For this review, take the finished solid that the model builds, in its own axes (mm). A direction names the side the tool comes from. Coordinates: 2 decimals unless noted, no trailing zeros. Order: outer loops, then holes, each group sorted by start corner. A loop starts at its lowest first (then second) coordinate and runs counter-clockwise, first axis right, second up.
from build123d import *

# Parameters (mm, degrees)
SKETCH1_R               = 4
BOSS_EXTRUDE1_DEPTH     = 3
SKETCH1_3_R             = 2.5
BOSS_EXTRUDE2_DEPTH     = 13
BOSS_EXTRUDE3_DEPTH     = 1.5
CUT_EXTRUDE1_DEPTH      = 15.177446879
CUT_EXTRUDE1_DEPTH_BACK = 15.177446879
SKETCH2_W               = 10
SKETCH2_H               = 3


with BuildPart() as part:
    # Sketch1 → Boss-Extrude1 (new body)
    with BuildSketch(Plane(origin=(0, 0, 0), x_dir=(0, 0, -1), z_dir=(1, 0, 0))):
        Circle(SKETCH1_R)
    extrude(amount=BOSS_EXTRUDE1_DEPTH)

    # Sketch1<3> → Boss-Extrude2 (add)
    with BuildSketch(Plane(origin=(0, 0, 0), x_dir=(0, 0, -1), z_dir=(1, 0, 0))):
        Circle(SKETCH1_3_R)
    extrude(amount=-BOSS_EXTRUDE2_DEPTH)

    # Sketch3 → Boss-Extrude3 (add, symmetric)
    with BuildSketch(Plane(origin=(0, 0, 0), x_dir=(1, 0, 0), z_dir=(0, 1, 0))):
        with BuildLine():
            Line((-11, 2.5), (-11, -2.5))
            ThreePointArc((-11, -2.5), (-12, -3.5), (-13, -2.5))
            Line((-13, -2.5), (-13, 2.5))
            ThreePointArc((-13, 2.5), (-12, 3.5), (-11, 2.5))
        make_face()
    extrude(amount=BOSS_EXTRUDE3_DEPTH, both=True)

    # Sketch2 → Cut-Extrude1 (cut, two sides: drawn at the far end of the back side and taken through both)
    with BuildSketch(Plane(origin=(0, 0, 0), x_dir=(1, 0, 0), z_dir=(0, 1, 0)).offset(-CUT_EXTRUDE1_DEPTH_BACK)):
        with Locations((-8, 0)):
            Rectangle(SKETCH2_W, SKETCH2_H)
    extrude(amount=CUT_EXTRUDE1_DEPTH + CUT_EXTRUDE1_DEPTH_BACK, mode=Mode.SUBTRACT)


solid = part.part
1. Take a section at D-D, the plane x = 0.75. Give the boundary of the cut face in (y, z).
Answer below:
outline: circle Ø8 at (0, 0)
2. Take a section at A-A, the plane x = -12. Give the boundary of the cut face in (y, z).
Answer below:
outline: (-2, -1.5) arc R2.5 ccw to (-1.5, -2) - (-1.5, -3.5) - (1.5, -3.5) - (1.5, -2) arc R2.5 ccw to (2, -1.5) - close; (-2, 1.5) - (2, 1.5) arc R2.5 ccw to (1.5, 2) - (1.5, 3.5) - (-1.5, 3.5) - (-1.5, 2) arc R2.5 ccw to start
3. Take a section at C-C, the plane z = -3. Give the boundary of the cut face in (x, y), plus the area to 3 significant figures.
Answer below:
outline: (-12.87, -1.5) - (-11.13, -1.5) - (-11.13, 1.5) - (-12.87, 1.5) - close; (0, -2.65) - (3, -2.65) - (3, 2.65) - (0, 2.65) - close
area: 21.1 mm2
4. The part is to be moulded in two halves that separate along X. For faces 1 (the face through (-8, 0, -1.5)), 2 (the face through (-12, 0, 3.5)), 3 (the face through (3, 0, 0)), say which applies: +X half, -X half, draft (parallel to the pull), parting line (faces both ways), or undercut.
Answer below:
face 1: draft
face 2: undercut
face 3: +X half
5. Take a section at B-B, the plane z = 0. Give the boundary of the cut face in (x, y), plus the area to 3 significant figures.
Answer below:
outline: (-3, -2.5) - (0, -2.5) - (0, -4) - (3, -4) - (3, 4) - (0, 4) - (0, 2.5) - (-3, 2.5) - close
area: 39.0 mm2
6. To check wall thickness, follow L1, parallel to X at y = 1.25, z = 2.5; L2, parallel to Z at x = -9.5, y = 0; L3, parallel to X at y = 3, z = -0.75. State the ranges of each line that lie inside material, in increasing order.
Answer below:
L1: x = -13 to -11, 0 to 3
L2: z = -2.5 to -1.5, 1.5 to 2.5
L3: x = 0 to 3
7. Machinability: for faces 4 (the face through (-12, 1.5, 3)), 5 (the face through (-8, 0, 1.5)), 6 (the face through (-12, -1.5, 3)), 7 (the face through (-12, 1.5, -3)), 8 (the face through (0, 2, -2)), which of the approach directions +Z, -Z, +X, -X, +Y, -Y give a long, thin tool a straight path to every point of the face, cutting with its end or side? Answer none if there is none.
Answer below:
face 4: +Z, -X, +Y
face 5: -X, +Y, -Y
face 6: +Z, -X, -Y
face 7: -Z, -X, +Y
face 8: none
8. Clearance check with flat-ended pins moving along their axes: pin 1 Ø1 at (x, y) = (1, -2.5) entering from +Z; pin 2 Ø1.7 at (x, z) = (-12, 3) entering from +Y; pin 3 Ø2 at (x, y) = (-9, 1) entering from +Z. State where each tip first meets the part, or that it passes through.
Answer below:
pin 1: stops at z = 3.46
pin 2: stops at y = 1.5
pin 3: stops at z = 2.5
